from build123d import *

# Parameters (mm, degrees)
F1_DEPTH = 58
F2_W     = 21.7170343468
F2_H     = 36
F2_W_2   = 18.1216797089
F2_W_3   = 101.6265741507
F3_DEPTH = 11
F5_DEPTH = 27
F6_DEPTH = 27
F7_R     = 5
F8_R     = 5


# Not quite as in the source:
# - a feature names something its author has since deleted; it is built from what else it names


with BuildPart() as f1:
    # F0 (on Front) → F1 (new body)
    with BuildSketch(Plane.XZ):
        with BuildLine():
            Line((0, 6), (0, 0))
            Line((0, 0), (105, 0))
            Line((105, 0), (105, 6))
            Line((105, 6), (116, 6))
            ThreePointArc((116, 6), (115.651030618, 23.7706667749), (105, 38))
            Line((105, 38), (3.3734258493, 38))
            ThreePointArc((3.3734258493, 38), (-0.1544899089, 37.3225666374), (-3.1805835495, 35.3866268563))
            ThreePointArc((-3.1805835495, 35.3866268563), (-11.2509687534, 21.8004179002), (-11, 6))
            Line((-11, 6), (0, 6))
        make_face()
    extrude(amount=-F1_DEPTH)

    # F2 (on face) → F3 (cut)
    with BuildSketch(Plane.XY.offset(38)):
        with Locations((115.8585171734, 29)):
            Rectangle(F2_W, F2_H)
        with Locations((-5.6874140052, 29)):
            Rectangle(F2_W_2, F2_H)
        with Locations((54.1867129246, 29)):
            Rectangle(F2_W_3, F2_H)
    extrude(amount=-F3_DEPTH, mode=Mode.SUBTRACT)

    # F4 (on face) → F5 (cut)
    with BuildSketch(Plane.XY.offset(27)):
        with BuildLine():
            Line((33, 35.5), (14, 35.5))
            ThreePointArc((14, 35.5), (7.5, 29), (14, 22.5))
            Line((14, 22.5), (33, 22.5))
            ThreePointArc((33, 22.5), (39.5, 29), (33, 35.5))
        make_face()
    extrude(amount=-F5_DEPTH, mode=Mode.SUBTRACT)

    # F4 (on face) → F6 (cut)
    with BuildSketch(Plane.XY.offset(27)):
        with BuildLine():
            Line((91, 35.5), (72, 35.5))
            ThreePointArc((72, 35.5), (65.5, 29), (72, 22.5))
            Line((72, 22.5), (91, 22.5))
            ThreePointArc((91, 22.5), (97.5, 29), (91, 35.5))
        make_face()
    extrude(amount=-F6_DEPTH, mode=Mode.SUBTRACT)

    # F7
    f7_edges = [f1.edges().sort_by_distance(p)[0] for p in [
        (54.186713, 0, 38),
        (115.651031, 0, 23.770667),
    ]]
    fillet(f7_edges, radius=F7_R)

    # F8
    f8_edges = [f1.edges().sort_by_distance(p)[0] for p in [
        (115.651031, 58, 23.770667),
        (54.186713, 58, 38),
    ]]
    fillet(f8_edges, radius=F8_R)


solid = f1.part
Geometry check sheet. Reference: the model listing, model coordinates, mm. A direction names the side the tool comes from. Give positions to 0.01 mm unless a question says otherwise; leave off trailing zeros. Write each loop counter-clockwise with the first axis right and the second up, starting at its lowest first coordinate (ties: lowest second). Pieces come first, ordered by that corner, then holes. Notation, with made-up numbers: (-5.75, 19) - (50.25, 19) arc R29 cw to (50.25, 54) - close; hole circle Ø11 at (85, -21). An arc over 180 degrees is marked (long way). Put each result on its own line as item: value.
1. Thickness scan on line 1 (X direction, y = 31, z = 26); line 2 (Y direction, x = 68, z = 33); line 3 (Y direction, x = 30.5, z = 7). Record the ranges inside material, lowest first.
Ans:
line 1: x = -9.78 to 7.82, 39.18 to 65.82, 97.18 to 114.78
line 2: y = 0 to 11, 47 to 58
line 3: y = 0 to 22.5, 35.5 to 58
2. Sectioned sample at D-D, the plane z = 12.5. Give the number of separate pieces and of enclosed holes in the cut face, plus the area to 3 significant figures.
Ans:
separate pieces: 1
enclosed holes: 2
area: 6,720 mm²
3. Go/stop test with flat-tipped pins: pin 1 (3 mm diameter, centred on x = 37.5, y = 19, fed in from +Z); pin 2 (5 mm diameter, centred on y = 25, z = 4, fed in from +X); pin 3 (3 mm diameter, centred on y = 42, z = 1.5, fed in from -X). Record where each tip stops, or that it passes through.
Ans:
pin 1: stops at z = 27
pin 2: stops at x = 116.15
pin 3: stops at x = 0
4. Sectioned sample at B-B, the plane x = 75.5. Enter the section's corners in (y, z), plus the area to 3 significant figures.
Ans:
outline: (0, 0) - (22.5, 0) - (22.5, 27) - (11, 27) - (11, 38) - (5, 38) arc R5 ccw to (0, 33) - close; (35.5, 0) - (58, 0) - (58, 33) arc R5 ccw to (53, 38) - (47, 38) - (47, 27) - (35.5, 27) - close
area: 1,450 mm²
5. Set-up check for faces 1 (the flat face through (23, 22.5, 14)), 2 (the flat face through (105, 29, 3)), 3 (the flat face through (52, 29, 27)), 4 (the flat face through (-6, 29, 6)): record each of +Z, -Z, +X, -X, +Y, -Y from which the full face is reachable in a straight line by a thin tool's end or side.
Ans:
face 1: +Z, -Z
face 2: -Z, +X, +Y, -Y
face 3: +Z, +X, -X
face 4: -Z, -X, +Y, -Y
6. Sectioned sample at A-A, the plane y = 29. Enter the section's corners in (x, z).
Ans:
outline: (-11, 6) - (0, 6) - (0, 0) - (7.5, 0) - (7.5, 27) - (-9.32, 27) arc R29 ccw to start; (39.5, 0) - (65.5, 0) - (65.5, 27) - (39.5, 27) - close; (97.5, 0) - (105, 0) - (105, 6) - (116, 6) arc R29 ccw to (114.32, 27) - (97.5, 27) - close
7. Sectioned sample at C-C, the plane y = 18. Enter the section's corners in (x, z), plus the area to 3 significant figures.
Ans:
outline: (-11, 6) - (0, 6) - (0, 0) - (105, 0) - (105, 6) - (116, 6) arc R29 ccw to (114.32, 27) - (-9.32, 27) arc R29 ccw to start
area: 3,320 mm²
8. Draft check along Y on faces 5 (the flat face through (55, 50, 38)), 6 (the cylindrical face through (7.5, 29.1, 13.7)), 7 (the flat face through (52, 58, 17)). Enter one of: +Y half, -Y half, draft (parallel to the pull), parting line (faces both ways), or undercut.
Ans:
face 5: draft
face 6: undercut
face 7: +Y half
